Study the drawing (mm; zero at the part's minimum x, y, z) and answer. Round coordinates to 2 decimals unless told otherwise and drop trailing zeros. Write each loop counter-clockwise with the first axis right and the second up, starting at its lowest first coordinate (ties: lowest second). Pieces come first, ordered by that corner, then holes. Notation, with made-up numbers: (78.5, 78.25) - (96.5, 78.25) arc R33 ccw to (96.5, 112.25) - close; hole circle Ø11 at (89, 62). An arc over 180 degrees is marked (long way). Return JSON: item names as keys, results as strings. Group by question number.
(1) Find the intervals of material crossed by line 1 along Y through (x, z) = (3, 6); line 2 along X through (y, z) = (13.5, 2.5); line 3 along Y through (x, z) = (11, 1.7), in increasing order. Write a range as [from, to].
(2) Section B-B, the plane z = 7 is taken. Write down the section's boundary in (x, y), then the cut area to 3 significant figures.
(3) Each of these flat-tipped pins is pushed along its axis until it touches: pin 1 (3.5 mm diameter, centred on x = 11, y = 13.8, fed in from -Z); pin 2 (5 mm diameter, centred on x = 31, y = 13.8, fed in from +Z). Where does it stop, or does it pass through?
(4) Section A-A, the plane y = 13.8 is taken. Write down the section's boundary in (x, z), then the cut area to 3 significant figures.
(5) Section D-D, the plane y = 3 is taken. Write down the section's boundary in (x, z).
(6) Section C-C, the plane x = 31 is taken. Write down the section's boundary in (y, z), then the cut area to 3 significant figures.
(7) Determine the mould class of the marked faces 1, 2 and 3 for opening direction Y: +Y half, -Y half, draft (parallel to the pull), parting line (faces both ways), or undercut.
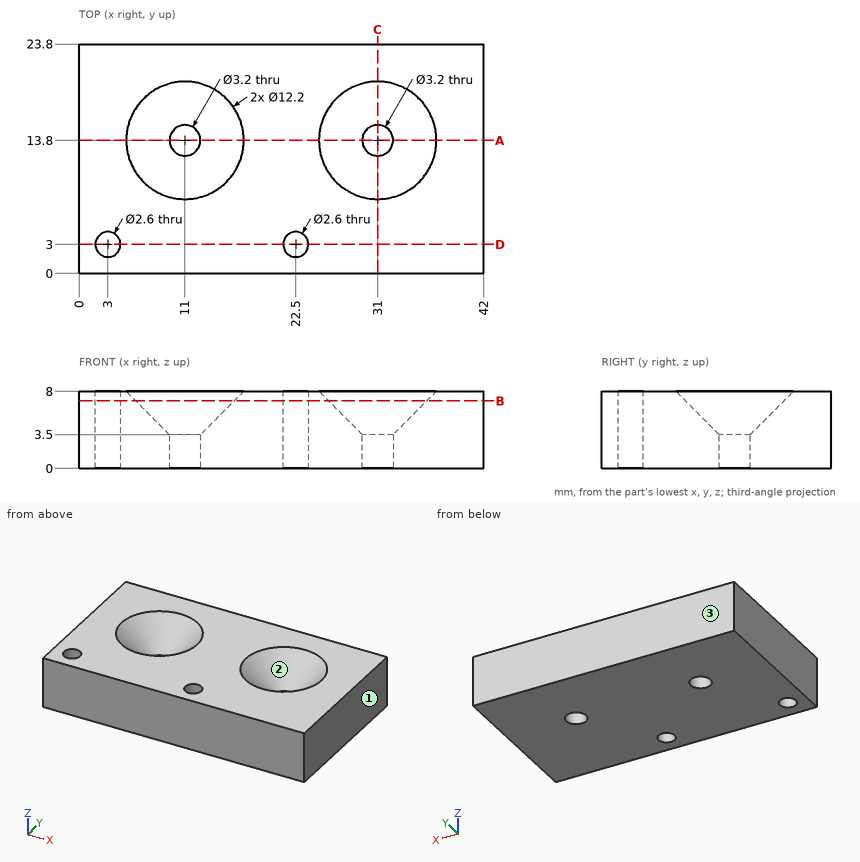
Working result:
{
 "1": {"line 1": "y = [0, 1.7], [4.3, 23.8]", "line 2": "x = [0, 9.43], [12.57, 29.43], [32.57, 42]", "line 3": "y = [0, 12.2], [15.4, 23.8]"},
 "2": {"outline": "(0, 0) - (42, 0) - (42, 23.8) - (0, 23.8) - close; hole circle Ø2.6 at (3, 3); hole circle Ø10.2 at (11, 13.8); hole circle Ø2.6 at (22.5, 3); hole circle Ø10.2 at (31, 13.8)", "area": "826 mm^2"},
 "3": {"pin 1": "stops at z = 0", "pin 2": "stops at z = 4.4"},
 "4": {"outline": "(0, 0) - (9.4, 0) - (9.4, 3.5) - (4.9, 8) - (0, 8) - close; (12.6, 0) - (29.4, 0) - (29.4, 3.5) - (24.9, 8) - (17.1, 8) - (12.6, 3.5) - close; (32.6, 0) - (42, 0) - (42, 8) - (37.1, 8) - (32.6, 3.5) - close", "area": "244 mm^2"},
 "5": {"outline": "(0, 0) - (1.7, 0) - (1.7, 8) - (0, 8) - close; (4.3, 0) - (21.2, 0) - (21.2, 8) - (4.3, 8) - close; (23.8, 0) - (42, 0) - (42, 8) - (23.8, 8) - close"},
 "6": {"outline": "(0, 0) - (12.2, 0) - (12.2, 3.5) - (7.7, 8) - (0, 8) - close; (15.4, 0) - (23.8, 0) - (23.8, 8) - (19.9, 8) - (15.4, 3.5) - close", "area": "145 mm^2"},
 "7": {"face 1": "draft", "face 2": "undercut", "face 3": "+Y half"}
}
